Autodesk Inventor part; units mm, degrees
ref_plane "YZ Plane" through (0, 0, 0) normal (1, 0, 0) x (0, 1, 0)
ref_plane "XZ Plane" through (0, 0, 0) normal (0, 1, 0) x (-1, 0, 0)
ref_plane "XY Plane" through (0, 0, 0) normal (0, 0, 1) x (1, 0, 0)
sketch "Sketch1" plane through (0, 0, 0) normal (0, 1, 0) x (-1, 0, 0)
  line L0 (0, 0) -> (16, 0)
  line L1 (16, 0) -> (16, -54)
  line L2 (16, -54) -> (0, -54)
  line L3 (0, -54) -> (0, 0)
  dimension "d0" = 16
  dimension "d1" = 54
extrude "Extrusion1" add sketch "Sketch1" along normal blind 4.5
sketch "Sketch2" plane through (0, 4.5, 0) normal (0, 1, 0) x (1, 0, 0)
  line L0 (-16, 0) -> (0, 0)
  line L1 (0, 0) -> (0, 54)
  line L2 (0, 54) -> (-16, 54)
  line L3 (-16, 54) -> (-16, 0)
  line L4 (-16, 0) -> (0, 0)
  line L5 (0, 0) -> (0, 54)
  line L6 (-16, 0) -> (0, 54) construction
  line L7 (-16, 54) -> (-16, 0) construction
  line L8 (-16, 54) -> (0, 0) construction
  point P0 (-8, 27)
  point P1 (-8, 27)
hole "Hole1" at (-8, 4.5, -27) direction (0, -1, 0) diameter 10 end through all
chamfer "Chamfer1" distance 0.2 angle 45 2 edges at (-8, 0, -32) (-8, 4.5, -32)
sketch "Sketch3" plane through (0, 4.5, 0) normal (0, 1, 0) x (1, 0, 0)
  line L0 (0, 38) -> (-16, 38) construction
  line L1 (-16, 38) -> (-16, 54) construction
  line L2 (-16, 54) -> (0, 54) construction
  line L3 (0, 54) -> (0, 38) construction
  line L4 (0, 38) -> (-16, 54) construction
  line L5 (-16, 38) -> (0, 54) construction
  line L6 (-2.5, 51.5) -> (-13.5, 51.5) construction
  line L7 (-13.5, 51.5) -> (-13.5, 40.5) construction
  line L8 (-13.5, 40.5) -> (-2.5, 40.5) construction
  line L9 (-2.5, 40.5) -> (-2.5, 51.5) construction
  line L10 (-2.5, 51.5) -> (-13.5, 40.5) construction
  line L11 (-13.5, 51.5) -> (-2.5, 40.5) construction
  line L12 (0, 54) -> (-16, 54) construction
  line L13 (-16, 54) -> (-16, 0) construction
  line L14 (-16, 0) -> (0, 0) construction
  line L15 (0, 0) -> (0, 54) construction
  circle A0 centre (-8, 27) radius 5.2 construction
  line L16 (-16, 27) -> (0, 27) construction
  point P0 (-8, 46)
  point P1 (-2.5, 13.5)
  point P2 (-13.5, 13.5)
  point P3 (-13.5, 2.5)
  point P4 (-2.5, 2.5)
  dimension "d16" = 16
  dimension "d17" = 16
  dimension "d18" = 11
  dimension "d19" = 11
hole "Hole2" at (-2.5, 4.5, -40.5) at (-13.5, 4.5, -40.5) at (-13.5, 4.5, -51.5) at (-2.5, 4.5, -51.5) at (-13.5, 4.5, -2.5) at (-13.5, 4.5, -13.5) at (-2.5, 4.5, -13.5) at (-2.5, 4.5, -2.5) direction (0, -1, 0) diameter 1.1835 end through all
chamfer "Chamfer2" distance 0.2 angle 45 8 edges at (-2.5, 4.5, -52.0917) (-2.5, 4.5, -41.0917) (-13.5, 4.5, -52.0917) (-13.5, 4.5, -41.0917) (-2.5, 4.5, -14.0917) (-2.5, 4.5, -3.0917) (-13.5, 4.5, -14.0917) (-13.5, 4.5, -3.0917)
properties part number "KN-00-02-01" material "X5CrNi18-10"
Design review of the part built by this model. Coordinates are the model's own, in mm. Give positions to 0.01 mm unless a question says otherwise; leave off trailing zeros. Loops run counter-clockwise (first coordinate to the right, second up) from the corner with the lowest first, then second, coordinate; pieces in that order, holes last. Notation, with made-up numbers: M -10.5,69 L 42.5,69 A32 cw 42.5,101 Z; hole C 65.25,-21 d3. An arc over 180 degrees is marked long. Return JSON: item names as keys, results as strings. Group by question number.
Item 1: For probe 1 along Z at (x, y) = (-2.5, 2.5); probe 2 along X at (y, z) = (3.1, -40.5); probe 3 along X at (y, z) = (1.45, -51), list the stretches that pass through material, from the lowest coordinate up.
Item 2: Mouldability with a two-part tool opening along X and no side actions: class faces 1 (the flat face through (0, 2, -27)), 2 (the flat face through (-16, 2, -27)), 3 (the flat face through (-8, 4.5, -33)), 4 (the cylindrical face through (-12.975, 2.12, -51.227)) as released by +X, released by -X, zero draft, split by the parting line, or undercut.
Item 3: We need section D-D (z = -2.5). Give the boundary of the cut face in (x, y), and give its area (3 significant figures).
Item 4: We need section B-B (z = -27). Give the boundary of the cut face in (x, y).
Item 5: We need section C-C (y = 1.2). Give the number of separate pieces and of enclosed holes in the cut face, and give its area (3 significant figures).
Item 6: We need section A-A (x = -8). Give the boundary of the cut face in (y, z), and give its area (3 significant figures).
Item 7: Insertion check: pin 1 Ø1.5 at (y, z) = (0.5, -20) entering from +X; pin 2 Ø0.7 at (x, z) = (-2.5, -51.5) entering from +Y; pin 3 Ø1.4 at (x, z) = (-13.5, -40.5) entering from +Y; pin 4 Ø1.5 at (x, z) = (-13.5, -51.5) entering from +Y. Each pin has a flat end and moves straight along its axis. Give the tip position at first contact, or say it passes through.
Output:
{
 "1": {"probe 1": "z = -54 to -52.09, -50.91 to -41.09, -39.91 to -14.09, -12.91 to -3.09, -1.91 to 0", "probe 2": "x = -16 to -14.09, -12.91 to -3.09, -1.91 to 0", "probe 3": "x = -16 to -13.82, -13.18 to -2.82, -2.18 to 0"},
 "2": {"face 1": "released by +X", "face 2": "released by -X", "face 3": "zero draft", "face 4": "undercut"},
 "3": {"outline": "M -16,0 L -14.09,0 L -14.09,4.3 L -14.29,4.5 L -16,4.5 Z; M -12.91,0 L -3.09,0 L -3.09,4.3 L -3.29,4.5 L -12.71,4.5 L -12.91,4.3 Z; M -1.91,0 L 0,0 L 0,4.5 L -1.71,4.5 L -1.91,4.3 Z", "area": "61.3 mm^2"},
 "4": {"outline": "M -16,0 L -13.2,0 L -13,0.2 L -13,4.3 L -13.2,4.5 L -16,4.5 Z; M -3,0.2 L -2.8,0 L 0,0 L 0,4.5 L -2.8,4.5 L -3,4.3 Z"},
 "5": {"separate pieces": "1", "enclosed holes": "9", "area": "777 mm^2"},
 "6": {"outline": "M 0,-54 L 4.5,-54 L 4.5,-32.2 L 4.3,-32 L 0.2,-32 L 0,-32.2 Z; M 0,-21.8 L 0.2,-22 L 4.3,-22 L 4.5,-21.8 L 4.5,0 L 0,0 Z", "area": "198 mm^2"},
 "7": {"pin 1": "stops at x = 0", "pin 2": "passes through", "pin 3": "stops at y = 4.41", "pin 4": "stops at y = 4.46"}
}
